from build123d import *

# Parameters (mm, degrees)
SKETCH2_W                                       = 584.2
SKETCH2_H                                       = 1727.2
BOSS_EXTRUDE1_DEPTH                             = 6.35
CUT_EXTRUDE1_DEPTH                              = 7.35
H_0_266_DIAMETER_HOLE1_D                        = 6.7564
FILLET1_R                                       = 6.35
SKETCH7_R                                       = 3.96875
CUT_EXTRUDE2_DEPTH                              = 12.7
CSK_FOR_10_FLAT_HEAD_MACHINE_SCREW1_D           = 5.6134
CSK_FOR_10_FLAT_HEAD_MACHINE_SCREW1_CSINK_D     = 9.779
CSK_FOR_10_FLAT_HEAD_MACHINE_SCREW1_CSINK_ANGLE = 82
SKETCH15_R                                      = 3.937
CUT_EXTRUDE3_DEPTH                              = 7.35
F_5_16_0_3125_DIAMETER_HOLE1_D                  = 7.9375


with BuildPart() as part:
    # Sketch2 → Boss-Extrude1 (new body)
    with BuildSketch(Plane.XY):
        with Locations((292.1, 863.6)):
            Rectangle(SKETCH2_W, SKETCH2_H)
    extrude(amount=BOSS_EXTRUDE1_DEPTH)

    # Sketch3 → Cut-Extrude1 (cut, through all)
    with BuildSketch(Plane.XY.offset(6.35)):
        Polygon((584.2, 1098.55), (311.15, 1098.55), (311.15, 184.15), (431.8, 63.5), (431.8, 0), (584.2, 0), align=None)
    extrude(amount=-CUT_EXTRUDE1_DEPTH, mode=Mode.SUBTRACT)

    # H (0.266) Diameter Hole1 (through all)
    with Locations(Plane.XY.offset(6.35)):
        with Locations((12.7, 1714.5), (12.7, 1289.05), (12.7, 863.6), (12.7, 438.15), (12.7, 12.7), (571.5, 1111.25), (571.5, 1412.875), (571.5, 1714.5)):
            Hole(H_0_266_DIAMETER_HOLE1_D / 2)

    # Fillet1
    fillet1_edges = [part.edges().sort_by_distance(p)[0] for p in [
        (431.8, 0, 3.175),
        (431.8, 63.5, 3.175),
        (311.15, 184.15, 3.175),
        (311.15, 1098.55, 3.175),
        (0, 0, 3.175),
    ]]
    fillet(fillet1_edges, radius=FILLET1_R)

    # Sketch7 → Cut-Extrude2 (cut)
    with BuildSketch(Plane.XY.offset(6.35)):
        with Locations((88.9, 12.7)):
            Circle(SKETCH7_R)
        with Locations((342.9, 12.7)):
            Circle(SKETCH7_R)
    extrude(amount=-CUT_EXTRUDE2_DEPTH, mode=Mode.SUBTRACT)

    # CSK for #10 Flat Head Machine Screw1 (through all)
    with Locations(Plane(origin=(0, 0, 0), x_dir=(-1, 0, 0), z_dir=(0, 0, -1))):
        with Locations((-304.8, 342.9), (-304.8, 215.9), (-320.317182668, 166.002561211), (-410.119743879, 76.2)):
            CounterSinkHole(CSK_FOR_10_FLAT_HEAD_MACHINE_SCREW1_D / 2, CSK_FOR_10_FLAT_HEAD_MACHINE_SCREW1_CSINK_D / 2, counter_sink_angle=CSK_FOR_10_FLAT_HEAD_MACHINE_SCREW1_CSINK_ANGLE)

    # Sketch15 → Cut-Extrude3 (cut, through all)
    with BuildSketch(Plane.XY.offset(6.35)):
        with Locations((378.46762, 19.05)):
            Circle(SKETCH15_R)
        with Locations((378.46762, 76.2)):
            Circle(SKETCH15_R)
    extrude(amount=-CUT_EXTRUDE3_DEPTH, mode=Mode.SUBTRACT)

    # 5/16 (0.3125) Diameter Hole1 (through all)
    with Locations(Plane(origin=(0, 0, 0), x_dir=(-1, 0, 0), z_dir=(0, 0, -1))):
        with Locations((-296.8625, 68.2625), (-296.8625, 14.2875)):
            Hole(F_5_16_0_3125_DIAMETER_HOLE1_D / 2)


solid = part.part
The listing builds one solid part. Answer for the finished solid, in the listing's coordinates (mm). Coordinates: 2 decimals unless noted, no trailing zeros. Loops run counter-clockwise (first coordinate to the right, second up) from the corner with the lowest first, then second, coordinate; pieces in that order, holes last. Notation, with made-up numbers: (89.25, 46) -> (97.25, 46) arc R32 cw to (97.25, 75) -> close; hole circle Ø10 at (21, -40). An arc over 180 degrees is marked (long way). Answer in a Markdown table with one row per item. Add a question column.
1. The part is cut by section C-C, the plane y = 615. Write down the section's boundary in (x, z).
2. Consider line 1 (X direction, y = 1714.5, z = 3); line 2 (Y direction, x = 304.8, z = 3.25); line 3 (Y direction, x = 12.7, z = 3). Determine where each line is inside the solid, lowest interval first. Write a range as [from, to].
3. Determine the mould class of faces 1 (the flat face through (370.7, 124.6, 3.2)), 2 (the flat face through (223, 1068, 0)) for opening direction Y: +Y half, -Y half, draft (parallel to the pull), parting line (faces both ways), or undercut.
4. The part is cut by section B-B, the plane x = 490.5. Write down the section's boundary in (y, z), then the cut area to 3 significant figures.
5. The part is cut by section A-A, the plane z = 5.25. Count the separate pieces of the cut face and the enclosed holes in it, then the cut area to 3 significant figures.
6. A flat-ended cylindrical pin translates along its axis: P1, Ø1.9, axis at y = 644, z = 4.5, coming from the +X side. Find the tip coordinate at first contact, or state that the pin passes through.
Answer below:
| question | item | result |
|---|---|---|
| 1 | outline | (0, 0) -> (311.15, 0) -> (311.15, 6.35) -> (0, 6.35) -> close |
| 2 | line 1 | [0, 9.32], [16.08, 568.12], [574.88, 584.2] |
| 2 | line 2 | [0, 213.09], [218.71, 340.09], [345.71, 1727.2] |
| 2 | line 3 | [0, 9.32], [16.08, 434.77], [441.53, 860.22], [866.98, 1285.67], [1292.43, 1711.12], [1717.88, 1727.2] |
| 3 | face 1 | undercut |
| 3 | face 2 | draft |
| 4 | outline | (1098.55, 0) -> (1727.2, 0) -> (1727.2, 6.35) -> (1098.55, 6.35) -> close |
| 4 | area | 3,990 mm2 |
| 5 | separate pieces | 1 |
| 5 | enclosed holes | 18 |
| 5 | area | 723,000 mm2 |
| 6 | P1 | x = 311.15 |
